For this review, take the finished solid that the model builds, in its own axes (mm). Coordinates: 2 decimals unless noted, no trailing zeros. Loops run counter-clockwise (first coordinate to the right, second up) from the corner with the lowest first, then second, coordinate; pieces in that order, holes last. Notation, with made-up numbers: (35.5, 15.25) - (69.5, 15.25) arc R13 cw to (69.5, 25.25) - close; hole circle Ø7 at (54, -17.75). An arc over 180 degrees is marked (long way). One line per item, written item: value. Start each with the question number.
1. To check wall thickness, follow line 1 (Z direction, x = 0, y = 14); line 2 (Z direction, x = -52, y = 21.75); line 3 (X direction, y = 8.75, z = 29.5). State the ranges of each line that lie inside material, in increasing order. Write a range as from..to.
2. Take a section at A-A, the plane x = 0. State the section outline as (y, z) points, and give its area (3 significant figures).
3. Take a section at C-C, the plane x = 69. State the section outline as (y, z) points.
4. Take a section at D-D, the plane y = 9. Count the separate pieces of the cut face and the enclosed holes in it, and give its area (3 significant figures).
5. The part is to be moulded in two halves that separate along Z. For faces 1 (the face through (37.193, 11.397, 51.266)), 2 (the face through (18, 22.479, 49)), 3 (the face through (-43.68, 11.08, -68.5)), say which applies: released by +Z, released by -Z, zero draft, split by the parting line, or undercut.
6. Take a section at B-B, the plane z = 0. State the section outline as (x, y) points, and give its area (3 significant figures).
7. Insertion check: pin 1 (6 mm diameter, centred on y = 17.5, z = 36.5, fed in from +X); pin 2 (23.5 mm diameter, centred on x = 66.41, z = 0, fed in from -Y); pin 3 (4 mm diameter, centred on y = 2.5, z = 49, fed in from +X); pin 4 (3 mm diameter, centred on y = 13, z = 14.5, fed in from +X). Each pin has a flat end and moves straight along its axis. Give the tip position at first contact, or say it passes through.
Autodesk Inventor part; units mm, degrees
ref_plane "YZ Plane" through (0, 0, 0) normal (1, 0, 0) x (0, 1, 0)
ref_plane "XZ Plane" through (0, 0, 0) normal (0, 1, 0) x (-1, 0, 0)
ref_plane "XY Plane" through (0, 0, 0) normal (0, 0, 1) x (1, 0, 0)
sketch "Sketch1" plane through (0, 0, 0) normal (0, 1, 0) x (-1, 0, 0)
  circle A0 centre (0, 0) radius 51.5874
  circle A1 centre (0, 0) radius 81.2419
  dimension "d0" = 103.1748
  dimension "d1" = 162.4838
extrude "Extrusion1" add sketch "Sketch1" along normal blind 22.479
sketch "Sketch2" plane through (0, 22.479, 0) normal (0, 1, 0) x (1, 0, 0)
  circle A0 centre (66.4146, 0) radius 7.4136
  circle A1 centre (57.5168, 33.2073) radius 7.4136
  circle A2 centre (33.2073, 57.5168) radius 7.4136
  circle A3 centre (0, 66.4146) radius 7.4136
  circle A4 centre (-33.2073, 57.5168) radius 7.4136
  circle A5 centre (-57.5168, 33.2073) radius 7.4136
  circle A6 centre (-66.4146, 0) radius 7.4136
  circle A7 centre (-57.5168, -33.2073) radius 7.4136
  circle A8 centre (-33.2073, -57.5168) radius 7.4136
  circle A9 centre (0, -66.4146) radius 7.4136
  circle A10 centre (33.2073, -57.5168) radius 7.4136
  circle A11 centre (57.5168, -33.2073) radius 7.4136
  point P0 (0, 0)
  dimension "d4" = 14.8272
  dimension "d6" = 66.4146
  dimension "d9" = 360
extrude "Extrusion2" cut sketch "Sketch2" against normal through all
equation "\"d0\" = insideDiam"
equation "\"d1\" = outsideDiam"
equation "\"d2\" = thickness"
equation "\"d4\" = stregthenHoleDiam"
equation "\"d11\" = thickness"
equation "\"thickness\" = 22.479"
equation "\"printerError\" = 0.508"
equation "\"shellWidth\" = -0.5 * insideDiam + 0.5 * outsideDiam"
equation "\"stregthenHoleDiam\" = 0.5 * shellWidth"
equation "\"shellRadius\" = 0.5 * outsideDiam - 0.5 * shellWidth"
equation "\"numberOfHoles\" = 30.48"
properties part number "vexSupportRing"
Solutions:
1. line 1: -81.24..-73.83, -59..-51.59, 51.59..59, 73.83..81.24
1. line 2: -62.42..-38.16, -28.25..28.25, 38.16..62.42
1. line 3: -75.7..-63.94, -51.1..-42.32, 42.32..51.1, 63.94..75.7
2. outline: (0, -81.24) - (22.48, -81.24) - (22.48, -73.83) - (0, -73.83) - close; (0, -59) - (22.48, -59) - (22.48, -51.59) - (0, -51.59) - close; (0, 51.59) - (22.48, 51.59) - (22.48, 59) - (0, 59) - close; (0, 73.83) - (22.48, 73.83) - (22.48, 81.24) - (0, 81.24) - close
2. area: 667 mm2
3. outline: (0, -42.89) - (22.48, -42.89) - (22.48, -6.95) - (0, -6.95) - close; (0, 6.95) - (22.48, 6.95) - (22.48, 42.89) - (0, 42.89) - close
4. separate pieces: 1
4. enclosed holes: 13
4. area: 10,300 mm2
5. face 1: undercut
5. face 2: zero draft
5. face 3: split by the parting line
6. outline: (-81.24, 0) - (-73.83, 0) - (-73.83, 22.48) - (-81.24, 22.48) - close; (-59, 0) - (-51.59, 0) - (-51.59, 22.48) - (-59, 22.48) - close; (51.59, 0) - (59, 0) - (59, 22.48) - (51.59, 22.48) - close; (73.83, 0) - (81.24, 0) - (81.24, 22.48) - (73.83, 22.48) - close
6. area: 667 mm2
7. pin 1: x = 74.01
7. pin 2: y = 0
7. pin 3: x = 66.27
7. pin 4: x = 80.2
